Geometry: final body of the model. Coordinates: model frame, mm. Face numbers are marked on the shaded views. A direction names the side the tool comes from. Coordinates: 2 decimals unless noted, no trailing zeros. Loops run counter-clockwise (first coordinate to the right, second up) from the corner with the lowest first, then second, coordinate; pieces in that order, holes last. Notation, with made-up numbers: (48, -11) -> (80, -11) arc R27 ccw to (80, 11) -> close; hole circle Ø5 at (22, 7.25). An arc over 180 degrees is marked (long way). One line per item, written item: value. Start each with the question number.
Item 1: Section query D-D on y = -9. Return loops of the section in (x, z).
Item 2: Section query C-C on z = -0.5. Return loops of the section in (x, y), then the cut area to 3 significant figures.
Item 3: Section query B-B on x = 55.5. Return loops of the section in (y, z) (3 decimals).
Item 4: Section query A-A on y = -16.5. Return loops of the section in (x, z).
Item 5: Ray query, probe 1 along X at (y, z) = (-28, -2.75); probe 2 along X at (y, z) = (-19, 2.25); probe 3 along X at (y, z) = (-6, -4.5). Return the intervals inside material, ascending. Write a range as from..to.
Item 6: Set-up query: the marked faces 1, 2 and 3. Return all of +Z, -Z, +X, -X, +Y, -Y with unobstructed straight access to the full face (end or side cutting, diameter ignored); none if empty.
Item 7: Mould query, pull axis X, two halves, no side actions, for the marked faces 4, 5 and 6. Classes: +X half, -X half, draft (parallel to the pull), parting line (faces both ways), or undercut.
Item 8: Contact query for flat-ended pins moving along their axis: pin 1 Ø1 at (x, y) = (103.5, -21) entering from +Z; pin 2 Ø3 at (x, z) = (41, -1) entering from -Y; pin 3 Ø6 at (x, z) = (58.5, 6.5) entering from -Y; pin 4 Ø5.5 at (y, z) = (-11, -3) entering from -X. Output: stop coordinate, or through.
from build123d import *

# Parameters (mm, degrees)
SKETCH1_W           = 17.78
SKETCH1_H           = 6.35
BOSS_EXTRUDE1_DEPTH = 5.08
BOSS_EXTRUDE2_DEPTH = 50.8
SKETCH1_4_W         = 17.78
SKETCH1_4_H         = 6.35
BOSS_EXTRUDE3_DEPTH = 17.78


with BuildPart() as part:
    # Sketch1 → Boss-Extrude1 (new body)
    with BuildSketch(Plane(origin=(0, 0, 0), x_dir=(0, 0, -1), z_dir=(1, 0, 0))):
        with Locations((0, -28.575)):
            Rectangle(SKETCH1_W, SKETCH1_H)
        Polygon((-3.175, -11.43), (-8.89, -3.81), (-8.89, -25.4), (8.89, -25.4), (8.89, -3.81), (3.175, -11.43), align=None)
        Polygon((3.175, -11.43), (-3.175, -11.43), (-8.89, -3.81), (8.89, -3.81), align=None)
        Polygon((3.175, 11.43), (-3.175, 11.43), (-8.89, 3.81), (-8.89, -3.81), (8.89, -3.81), (8.89, 3.81), align=None)
    extrude(amount=BOSS_EXTRUDE1_DEPTH)

    # Sketch1_3 → Boss-Extrude2 (add)
    with BuildSketch(Plane(origin=(0, 0, 0), x_dir=(0, 0, -1), z_dir=(1, 0, 0))):
        Polygon((3.175, -11.43), (-3.175, -11.43), (-8.89, -3.81), (8.89, -3.81), align=None)
        Polygon((3.175, 11.43), (-3.175, 11.43), (-8.89, 3.81), (-8.89, -3.81), (8.89, -3.81), (8.89, 3.81), align=None)
    extrude(amount=BOSS_EXTRUDE2_DEPTH)

    # Sketch1_4 → Boss-Extrude3 (add)
    with BuildSketch(Plane(origin=(0, 0, 0), x_dir=(0, 0, -1), z_dir=(1, 0, 0))):
        with Locations((0, -28.575)):
            Rectangle(SKETCH1_4_W, SKETCH1_4_H)
    extrude(amount=-BOSS_EXTRUDE3_DEPTH)

    # Mirror1: part across plane


with BuildPart() as part_1:
    add(part.part)
    add(part.part.mirror(Plane(origin=(50.8, 0, 0), x_dir=(0, 0, 1), z_dir=(1, 0, 0))))


solid = part_1.part
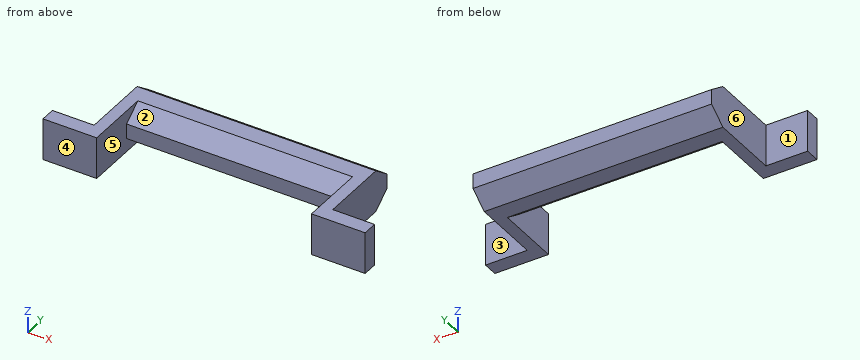
Reply:
1. outline: (0, -8.89) -> (5.08, -8.89) -> (5.08, -5) -> (96.52, -5) -> (96.52, -8.89) -> (101.6, -8.89) -> (101.6, 8.89) -> (96.52, 8.89) -> (96.52, 5) -> (5.08, 5) -> (5.08, 8.89) -> (0, 8.89) -> close
2. outline: (-17.78, -31.75) -> (5.08, -31.75) -> (5.08, -11.43) -> (96.52, -11.43) -> (96.52, -31.75) -> (119.38, -31.75) -> (119.38, -25.4) -> (101.6, -25.4) -> (101.6, 11.43) -> (0, 11.43) -> (0, -25.4) -> (-17.78, -25.4) -> close
2. area: 2,750 mm²
3. outline: (-11.43, -3.175) -> (-3.81, -8.89) -> (3.81, -8.89) -> (11.43, -3.175) -> (11.43, 3.175) -> (3.81, 8.89) -> (-3.81, 8.89) -> (-11.43, 3.175) -> close
4. outline: (0, -8.89) -> (5.08, -8.89) -> (5.08, 8.89) -> (0, 8.89) -> close; (96.52, -8.89) -> (101.6, -8.89) -> (101.6, 8.89) -> (96.52, 8.89) -> close
5. probe 1: x = -17.78..5.08, 96.52..119.38
5. probe 2: x = 0..5.08, 96.52..101.6
5. probe 3: x = 0..101.6
6. face 1: +Z, -Z, -X, +Y
6. face 2: +Z, -Y
6. face 3: +Z, -Z, +X, +Y
7. face 4: draft
7. face 5: undercut
7. face 6: -X half
8. pin 1: passes through
8. pin 2: stops at y = -11.43
8. pin 3: stops at y = -11
8. pin 4: stops at x = 0
